For this review, take the finished solid that the model builds, in its own axes (mm). Face numbers are marked on the shaded views. A direction names the side the tool comes from. Give positions to 0.01 mm unless a question says otherwise; leave off trailing zeros. Loops run counter-clockwise (first coordinate to the right, second up) from the corner with the lowest first, then second, coordinate; pieces in that order, holes last. Notation, with made-up numbers: (45, 22) - (67, 22) arc R11 ccw to (67, 28) - close; hole circle Ø9 at (44, 18). An arc over 180 degrees is marked (long way). Put each result on its own line as item: value.
from build123d import *

# Parameters (mm, degrees)
BOSS_EXTRUDE1_DEPTH = 20
SKETCH3_R           = 2
CUT_EXTRUDE1_DEPTH  = 6
SKETCH4_R           = 2
CUT_EXTRUDE2_DEPTH  = 6


with BuildPart() as part:
    # Sketch2 → Boss-Extrude1 (new body)
    with BuildSketch(Plane(origin=(0, 0, 0), x_dir=(0, 0, -1), z_dir=(1, 0, 0))):
        Polygon((-12.5, 0), (12.5, 0), (12.5, 25), align=None)
    extrude(amount=BOSS_EXTRUDE1_DEPTH)

    # Sketch3 → Cut-Extrude1 (cut)
    with BuildSketch(Plane(origin=(0, 0, -12.5), x_dir=(-1, 0, 0), z_dir=(0, 0, -1))):
        with Locations((-10, 10)):
            Circle(SKETCH3_R)
    extrude(amount=-CUT_EXTRUDE1_DEPTH, mode=Mode.SUBTRACT)

    # Sketch4 → Cut-Extrude2 (cut)
    with BuildSketch(Plane.XZ):
        with Locations(Location((10, -2.5, 0), (0, 0, 270))):
            Circle(SKETCH4_R)
    extrude(amount=-CUT_EXTRUDE2_DEPTH, mode=Mode.SUBTRACT)


solid = part.part
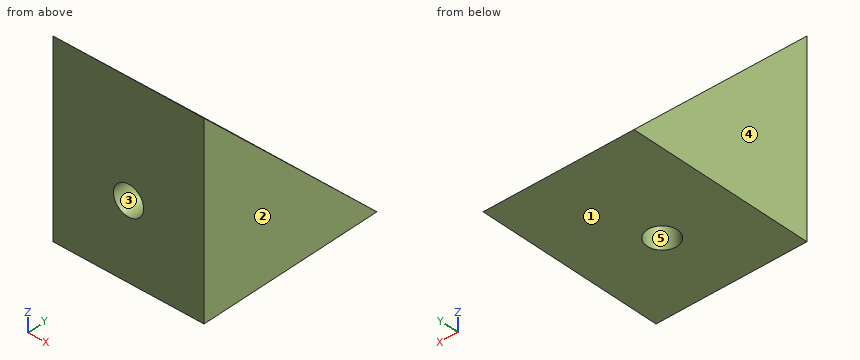
1) For the marked faces 4 and 5, list the 3-axis set-ups (+Z, -Z, +X, -X, +Y, -Y) from which the entire face can be reached by the end or side of a thin tool; tool diameter is ignored.
Geometry check:
face 4: +Z, -Z, -X, +Y, -Y
face 5: -Z
2) Take a section at B-B on x = 10. State the section outline as (y, z) points, and give its area (4 significant figures).
Geometry check:
outline: (0, -12.5) - (8, -12.5) - (8, -6.5) - (12, -6.5) - (12, -12.5) - (25, -12.5) - (0, 12.5) - (0, -0.5) - (6, -0.5) - (6, -4.5) - (0, -4.5) - close
area: 264.5 mm²
3) Take a section at A-A on z = -7.5. State the section outline as (x, y) points, and give its area (3 significant figures).
Geometry check:
outline: (0, 0) - (20, 0) - (20, 20) - (0, 20) - close; hole circle Ø4 at (10, 10)
area: 387 mm²
4) Insertion check: pin 1 Ø3.5 at (x, z) = (10, -2.5) entering from +Y; pin 2 Ø12 at (y, z) = (5, -3) entering from -X; pin 3 Ø3.5 at (x, y) = (10, 10) entering from -Z; pin 4 Ø2 at (x, y) = (10.5, 9) entering from +Z. Each pin has a flat end and moves straight along its axis. Give the tip position at first contact, or say it passes through.
Geometry check:
pin 1: stops at y = 16.75
pin 2: stops at x = 0
pin 3: stops at z = -6.5
pin 4: stops at z = 4.5
5) Wall thickness on line 1 (X direction, y = 3.75, z = -2.5); line 2 (X direction, y = 2.5, z = -3.5); line 3 (Y direction, x = 10, z = -10.8): over which ranges is each line inside the solid? List them lowest first.
Geometry check:
line 1: x = 0 to 8, 12 to 20
line 2: x = 0 to 8.27, 11.73 to 20
line 3: y = 0 to 8, 12 to 23.3
6) Take a section at D-D on z = -2.5. State the section outline as (x, y) points.
Geometry check:
outline: (0, 0) - (8, 0) - (8, 6) - (12, 6) - (12, 0) - (20, 0) - (20, 15) - (0, 15) - close
7) Draft analysis for pull direction Z (two halves, no side actions). For the marked faces 1, 2 and 3, state which applies: pulls with the +Z half, pulls with the -Z half, needs draft (parallel to the pull), parting line crosses it, or undercut.
Geometry check:
face 1: pulls with the -Z half
face 2: needs draft
face 3: undercut
8) Take a section at C-C on y = 10. State the section outline as (x, z) points, and give its area (3 significant figures).
Geometry check:
outline: (0, -12.5) - (8, -12.5) - (8, -6.5) - (12, -6.5) - (12, -12.5) - (20, -12.5) - (20, 2.5) - (0, 2.5) - close
area: 276 mm²
